Autodesk Inventor part; units mm, degrees
ref_plane "YZ Plane" through (0, 0, 0) normal (1, 0, 0) x (0, 1, 0)
ref_plane "XZ Plane" through (0, 0, 0) normal (0, 1, 0) x (-1, 0, 0)
ref_plane "XY Plane" through (0, 0, 0) normal (0, 0, 1) x (1, 0, 0)
sketch "Sketch1" plane through (0, 0, 0) normal (0, 0, 1) x (1, 0, 0)
  line L0 (0, 0) -> (70, 0)
  line L1 (70, 0) -> (70, 77.5)
  line L2 (70, 77.5) -> (0, 77.5)
  line L3 (0, 77.5) -> (0, 0)
  dimension "d0" = 70
  dimension "d1" = 77.5
extrude "Extrusion1" add sketch "Sketch1" along normal blind 95
sketch "Sketch3" plane through (0, 0, 95) normal (0, 0, 1) x (1, 0, 0)
  line L0 (0, 0) -> (70, 0)
  line L1 (70, 77.5) -> (0, 77.5)
  line L2 (70, 0) -> (35, 0)
  line L3 (35, 0) -> (35, 77.5)
  line L4 (35, 77.5) -> (70, 77.5)
  line L5 (70, 77.5) -> (70, 0)
extrude "Extrusion3" cut sketch "Sketch3" against normal through all
sketch "Sketch4" plane through (0, 77.5, 95) normal (0, 1, 0) x (1, 0, 0)
  line L0 (0, 95) -> (0, 0)
  line L1 (0, 0) -> (-12.5, 0)
  line L2 (35, 95) -> (0, 95)
  arc A0 (-12.5, 0) -> (0, 95) centre (-1145.4326, 197.3924) ccw
  line L3 (-12.5, -10) -> (35, -10) construction
  dimension "d9" = 1150
  dimension "d54" = 47.5
  dimension "d55" = 10
extrude "Extrusion4" add sketch "Sketch4" against normal blind 77.5
sketch "Sketch5" plane through (35, 0, 95) normal (1, 0, 0) x (0, 0, -1)
  line L0 (0, 77.5) -> (0, 86.25)
  line L1 (0, 0) -> (0, -8.75)
  line L2 (0, 0) -> (0, 77.5)
  line L3 (95, 77.5) -> (95, 0)
  arc A0 (0, 86.25) -> (95, 77.5) centre (152.8838, 1226.0423) ccw
  arc A1 (95, 0) -> (0, -8.75) centre (152.8838, -1148.5423) ccw
  line L4 (0, 77.5) -> (95, 77.5)
  line L5 (95, 0) -> (0, 0)
  line L6 (-10, 86.25) -> (-10, -8.75) construction
  point P0 (-10, 38.75)
  point P1 (0, 38.75)
  dimension "d14" = 1150
  dimension "d15" = 1150
  dimension "d52" = 10
  dimension "d53" = 95
extrude "Extrusion5" add sketch "Sketch5" against normal blind 55 contours L0 A0 L4 | L5 A1 L1
sketch "Sketch6" plane through (-20, 0, 0) normal (0, 1, 0) x (1, 0, 0)
  line L0 (20, 0) -> (0, 0)
  line L1 (0, -95) -> (0, 0)
  arc A0 (7.5, -95) -> (20, 0) centre (-1125.4326, 102.3924) ccw
  line L2 (7.5, -95) -> (0, -95)
extrude "Extrusion6" cut sketch "Sketch6" along normal through all both and the other way through all
fillet "Fillet3" radius 19 2 edges at (-5.299, 80.9203, 47.9253) (-5.299, -3.4203, 47.9253)
sketch "Sketch8" plane through (0, 0, 95) normal (0, 0, 1) x (1, 0, 0)
  line L0 (35, 86.25) -> (35, -8.75)
  line L1 (35, 77.5) -> (35, 0)
  circle A0 centre (35, 38.75) radius 35
  point P0 (0, 0)
  dimension "d23" = 70
extrude "Extrusion7" cut sketch "Sketch8" against normal blind 20
sketch "Sketch9" plane through (0, 0, 75) normal (0, 0, 1) x (1, 0, 0)
  line L0 (35, 73.75) -> (35, 3.75)
  circle A0 centre (35, 38.75) radius 15.5
  point P0 (0, 0)
  dimension "d26" = 31
extrude "Extrusion8" cut sketch "Sketch9" against normal blind 20
sketch "Sketch10" plane through (0, 0, 0) normal (0, 0, -1) x (-1, 0, 0)
  line L0 (-35, 77.5) -> (-35, 0)
  circle A0 centre (-35, 38.75) radius 12.5
  point P0 (0, 0)
  dimension "d29" = 25
extrude "Extrusion9" cut sketch "Sketch10" against normal blind 50
sketch "Sketch11" plane through (0, 0, 50) normal (0, 0, -1) x (-1, 0, 0)
  line L0 (-35, 26.25) -> (-35, 51.25)
  circle A0 centre (-35, 38.75) radius 2.5
  circle A1 centre (-26.5, 38.75) radius 2
  point P0 (0, 0)
  dimension "d32" = 5
  dimension "d33" = 4
  dimension "d34" = 8.5
extrude "Extrusion10" cut sketch "Sketch11" against normal through all
sketch "Sketch12" plane through (0, 0, 55) normal (0, 0, 1) x (1, 0, 0)
  circle A0 centre (26.5, 38.75) radius 2
  circle A1 centre (26.5, 38.75) radius 4.5
  point P0 (0, 0)
  dimension "d37" = 9
extrude "Extrusion11" cut sketch "Sketch12" against normal blind 3
sketch "Sketch14" plane through (0, 0, 50) normal (0, 0, -1) x (-1, 0, 0)
  arc A0 (-35, 36.25) -> (-35, 41.25) centre (-35, 38.75) ccw
  circle A1 centre (-35, 38.75) radius 4
  point P0 (0, 0)
  dimension "d40" = 8
extrude "Extrusion12" cut sketch "Sketch14" against normal blind 3
sketch "Sketch15" plane through (0, 0, 75) normal (0, 0, 1) x (1, 0, 0)
  arc A0 (35, 41.25) -> (35, 36.25) centre (35, 38.75) ccw
  circle A1 centre (10, 38.75) radius 2.5
  circle A2 centre (22.5, 17.0994) radius 2.5
  circle A3 centre (47.5, 17.0994) radius 2.5
  circle A4 centre (60, 38.75) radius 2.5
  circle A5 centre (47.5, 60.4006) radius 2.5
  circle A6 centre (22.5, 60.4006) radius 2.5
  point P0 (0, 0)
  dimension "d43" = 5
  dimension "d44" = 25
  dimension "d47" = 360
extrude "Extrusion13" cut sketch "Sketch15" against normal blind 25
sketch "Sketch17" plane through (35, 73.75, 95) normal (1, 0, 0) x (0, 0, -1)
  line L0 (90, -60) -> (55, -60)
  line L1 (55, -60) -> (55, -10)
  line L2 (55, -10) -> (90, -10)
  line L3 (90, -10) -> (90, -60)
  line L4 (95, -22.5) -> (95, -47.5)
  line L5 (0, 12.5) -> (95, 12.5)
  line L6 (95, 12.5) -> (95, -82.5)
  line L7 (95, -82.5) -> (0, -82.5)
  line L8 (0, -82.5) -> (0, 12.5)
  point P0 (95, -73.75)
  point P1 (90, -35)
  point P2 (95, -35)
  dimension "d62" = 35
  dimension "d63" = 50
  dimension "d64" = 5
extrude "Extrusion16" cut sketch "Sketch17" against normal through all
sketch "Sketch18" plane through (35, 13.75, 5) normal (1, 0, 0) x (0, 0, -1)
  line L0 (0, 4) -> (-8, 4)
  line L1 (-8, 4) -> (-8, 46)
  line L2 (-8, 46) -> (0, 46)
  line L3 (0, 46) -> (0, 4)
  line L4 (-35, 37.5) -> (-35, 12.5)
  line L5 (0, 12.5) -> (0, 37.5)
  point P0 (5, -13.75)
  point P1 (0, 25)
  dimension "d69" = 42
  dimension "d70" = 8
extrude "Extrusion17" cut sketch "Sketch18" against normal blind 25
sketch "Sketch19" plane through (35, 13.75, 5) normal (0, -1, 0) x (1, 0, 0)
  circle A0 centre (-15, 17.5) radius 2.5
  line L0 (0, 35) -> (0, 0)
  point P0 (-35, -5)
  point P1 (0, 17.5)
  dimension "d73" = 5
  dimension "d74" = 15
extrude "Extrusion18" cut sketch "Sketch19" against normal through all
sketch "Sketch20" plane through (35, 51.25, 40) normal (1, 0, 0) x (0, 0, -1)
  line L0 (35, -37.5) -> (35, -33.5)
  line L1 (0, 12.5) -> (35, 12.5)
  line L2 (35, 12.5) -> (35, -37.5)
  line L3 (35, -37.5) -> (0, -37.5)
  line L4 (0, -37.5) -> (0, 12.5)
  line L5 (34, 11.5) -> (1, 11.5)
  line L6 (1, 11.5) -> (1, -36.5)
  line L7 (1, -36.5) -> (34, -36.5)
  line L8 (34, -36.5) -> (34, 11.5)
  point P0 (40, -51.25)
  dimension "d77" = 1
extrude "Extrusion19" cut sketch "Sketch20" against normal through all
properties part number "AA016" material "ABS Plastic"
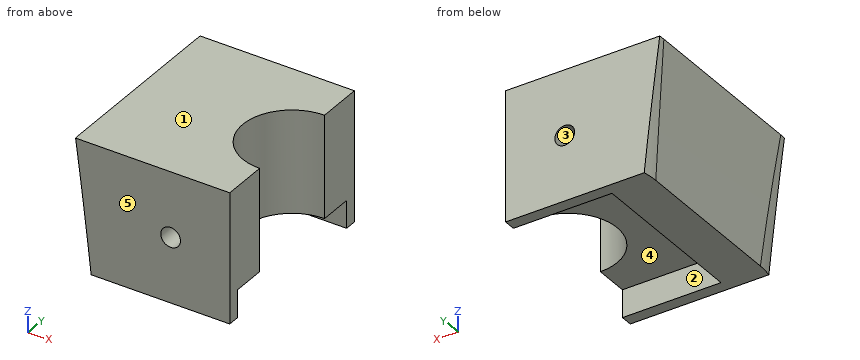
CAD build for the part. Positions are in the model's coordinates, mm. Face numbers are marked on the shaded views. A direction names the side the tool comes from. Round coordinates to 2 decimals unless told otherwise and drop trailing zeros. Loops run counter-clockwise (first coordinate to the right, second up) from the corner with the lowest first, then second, coordinate; pieces in that order, holes last. Notation, with made-up numbers: (31, 87) - (40, 87) arc R15 cw to (40, 103) - close; hole circle Ø1 at (-26, -34). An arc over 180 degrees is marked (long way). Return JSON: item names as keys, results as strings. Group by question number.
Q1. Flat gauge pins, fed straight in: pin 1 Ø3.5 at (y, z) = (35, 11) entering from +X; pin 2 Ø2 at (y, z) = (33.5, 18.5) entering from -X; pin 3 Ø1.5 at (y, z) = (46, 23) entering from -X; pin 4 Ø7.5 at (x, y) = (27, 37) entering from -Z. Where does each tip first touch, or does it go through?
Q2. Band-saw the part on C-C on x = 24.5. Give the cut face in (y, z), plus the area to 3 significant figures.
Q3. Drill centre lines: line 1 along Z through (x, y) = (20, 42.5); line 2 along Y through (x, z) = (29.5, 8); line 3 along Y through (x, z) = (31, 27.5). Where is each one in solid material? Low to high. Write a range as [from, to].
Q4. Tool access for the marked faces 1 and 2: list every direction of +Z, -Z, +X, -X, +Y, -Y with a clear straight run to the whole face (end or side of a thin tool).
Q5. Band-saw the part on D-D on y = 49.5. Give the cut face in (x, z).
Q6. Band-saw the part on B-B on y = 38.75. Give the cut face in (x, z), plus the area to 3 significant figures.
Q7. Band-saw the part on A-A on x = 20. Give the cut face in (y, z).
Q8. Two-plate mould, pull along Y, no slides. Class the marked faces 3, 4 and 5: +Y half, -Y half, draft (parallel to the pull), parting line (faces both ways), or undercut.
Solutions:
{
 "1": {"pin 1": "stops at x = 10", "pin 2": "stops at x = -1.91", "pin 3": "stops at x = -2.37", "pin 4": "passes through"},
 "2": {"outline": "(14.75, 6) - (17.75, 6) - (17.75, 13) - (31.97, 13) - (31.97, 39) - (14.75, 39) - close; (45.53, 13) - (59.75, 13) - (59.75, 6) - (62.75, 6) - (62.75, 39) - (45.53, 39) - close", "area": "937 mm^2"},
 "3": {"line 1": "z = [13, 20], [25, 39]", "line 2": "y = [14.75, 17.75], [59.75, 62.75]", "line 3": "y = [14.75, 26.91], [50.59, 62.75]"},
 "4": {"face 1": "+Z, +X, -X, +Y, -Y", "face 2": "-Z, +X"},
 "5": {"outline": "(-4.16, 39) arc R1150 cw to (-0.55, 6) - (10, 6) - (10, 13) - (28.62, 13) - (28.62, 39) - close; hole circle Ø5 at (20, 22.5)"},
 "6": {"outline": "(-4.16, 39) arc R1150 cw to (-0.55, 6) - (10, 6) - (10, 13) - (22.5, 13) - (22.5, 39) - close; hole circle Ø5 at (20, 22.5)", "area": "710 mm^2"},
 "7": {"outline": "(14.75, 6) - (17.75, 6) - (17.75, 13) - (59.75, 13) - (59.75, 6) - (62.75, 6) - (62.75, 20) - (14.75, 20) - close; (14.75, 25) - (62.75, 25) - (62.75, 39) - (14.75, 39) - close"},
 "8": {"face 3": "draft", "face 4": "undercut", "face 5": "-Y half"}
}
